Here's how the part is built. I have some questions about the finished solid (model axes, mm). Give positions to 0.01 mm unless a question says otherwise; leave off trailing zeros. Loops run counter-clockwise (first coordinate to the right, second up) from the corner with the lowest first, then second, coordinate; pieces in that order, holes last. Notation, with made-up numbers: (67.5, 26) - (119.5, 26) arc R21 cw to (119.5, 38) - close; hole circle Ø9 at (56, 71.5). An arc over 180 degrees is marked (long way). Return JSON: item names as keys, results as strings. Group by question number.
(1) If we section it at A-A (x = 149): Please give me the cut outline in (y, z) (1 decimal), then the cut area to 3 significant figures.
(2) I need wall thicknesses on probe 1 along X at (y, z) = (0.25, -214); probe 2 along Z at (x, y) = (221.5, -2). Which ranges of each line are inside material? Lowest first, please. Write a range as [from, to].
(3) If we section it at C-C (y = -0.5): State how many separate pieces and enclosed holes the cut face has, then the cut area to 3 significant figures.
(4) If we section it at B-B (z = -136): Please give me the cut outline in (x, y) (1 decimal), then the cut area to 3 significant figures.
```python
from build123d import *

# Parameters (mm, degrees)
SKETCH1_W                              = 382.775
SKETCH1_H                              = 356.150000032
BOSS_EXTRUDE1_DEPTH                    = 3.175
OUTER_SIDE_WALL_WELD_TAB_CUTOUTS_DEPTH = 6.35
CUT_EXTRUDE2_DEPTH                     = 6.35
CUT_EXTRUDE3_DEPTH                     = 6.35


with BuildPart() as part:
    # Sketch1 → Boss-Extrude1 (new body, symmetric)
    with BuildSketch(Plane(origin=(0, 0, 0), x_dir=(1, 0, 0), z_dir=(0, 1, 0))):
        with Locations((158.05, 144.737500016)):
            Rectangle(SKETCH1_W, SKETCH1_H)
    extrude(amount=BOSS_EXTRUDE1_DEPTH, both=True)

    # Sketch3 → Outer Side Wall Weld Tab Cutouts (cut)
    with BuildSketch(Plane(origin=(0, -3.175, 0), x_dir=(1, 0, 0), z_dir=(0, 1, 0))):
        with BuildLine():
            Line((314.5125, 53.318750008), (314.5125, 91.418750008))
            ThreePointArc((314.5125, 91.418750008), (316.1, 93.006250008), (317.6875, 91.418750008))
            Line((317.6875, 91.418750008), (317.6875, 53.318750008))
            ThreePointArc((317.6875, 53.318750008), (316.1, 51.731250008), (314.5125, 53.318750008))
        make_face()
        with BuildLine():
            Line((-1.5875, 53.318750008), (-1.5875, 91.418750008))
            ThreePointArc((-1.5875, 91.418750008), (0, 93.006250008), (1.5875, 91.418750008))
            Line((1.5875, 91.418750008), (1.5875, 53.318750008))
            ThreePointArc((1.5875, 53.318750008), (0, 51.731250008), (-1.5875, 53.318750008))
        make_face()
        with BuildLine():
            Line((314.5125, 125.687500016), (314.5125, 163.787500016))
            ThreePointArc((314.5125, 163.787500016), (316.1, 165.375000016), (317.6875, 163.787500016))
            Line((317.6875, 163.787500016), (317.6875, 125.687500016))
            ThreePointArc((317.6875, 125.687500016), (316.1, 124.100000016), (314.5125, 125.687500016))
        make_face()
        with BuildLine():
            Line((314.5125, 198.056250024), (314.5125, 236.156250024))
            ThreePointArc((314.5125, 236.156250024), (316.1, 237.743750024), (317.6875, 236.156250024))
            Line((317.6875, 236.156250024), (317.6875, 198.056250024))
            ThreePointArc((317.6875, 198.056250024), (316.1, 196.468750024), (314.5125, 198.056250024))
        make_face()
        with BuildLine():
            Line((-1.5875, 125.687500016), (-1.5875, 163.787500016))
            ThreePointArc((-1.5875, 163.787500016), (0, 165.375000016), (1.5875, 163.787500016))
            Line((1.5875, 163.787500016), (1.5875, 125.687500016))
            ThreePointArc((1.5875, 125.687500016), (0, 124.100000016), (-1.5875, 125.687500016))
        make_face()
        with BuildLine():
            Line((-1.5875, 198.056250024), (-1.5875, 236.156250024))
            ThreePointArc((-1.5875, 236.156250024), (0, 237.743750024), (1.5875, 236.156250024))
            Line((1.5875, 236.156250024), (1.5875, 198.056250024))
            ThreePointArc((1.5875, 198.056250024), (0, 196.468750024), (-1.5875, 198.056250024))
        make_face()
    extrude(amount=OUTER_SIDE_WALL_WELD_TAB_CUTOUTS_DEPTH, mode=Mode.SUBTRACT)

    # Sketch4 → Cut-Extrude2 (cut)
    with BuildSketch(Plane(origin=(0, -3.175, 0), x_dir=(1, 0, 0), z_dir=(0, 1, 0))):
        with BuildLine():
            Line((156.4625, 53.318750008), (156.4625, 91.418750008))
            ThreePointArc((156.4625, 91.418750008), (158.05, 93.006250008), (159.6375, 91.418750008))
            Line((159.6375, 91.418750008), (159.6375, 53.318750008))
            ThreePointArc((159.6375, 53.318750008), (158.05, 51.731250008), (156.4625, 53.318750008))
        make_face()
        with BuildLine():
            Line((77.4375, 53.318750008), (77.4375, 91.418750008))
            ThreePointArc((77.4375, 91.418750008), (79.025, 93.006250008), (80.6125, 91.418750008))
            Line((80.6125, 91.418750008), (80.6125, 53.318750008))
            ThreePointArc((80.6125, 53.318750008), (79.025, 51.731250008), (77.4375, 53.318750008))
        make_face()
        with BuildLine():
            Line((235.4875, 53.318750008), (235.4875, 91.418750008))
            ThreePointArc((235.4875, 91.418750008), (237.075, 93.006250008), (238.6625, 91.418750008))
            Line((238.6625, 91.418750008), (238.6625, 53.318750008))
            ThreePointArc((238.6625, 53.318750008), (237.075, 51.731250008), (235.4875, 53.318750008))
        make_face()
        with BuildLine():
            Line((156.4625, 125.687500016), (156.4625, 163.787500016))
            ThreePointArc((156.4625, 163.787500016), (158.05, 165.375000016), (159.6375, 163.787500016))
            Line((159.6375, 163.787500016), (159.6375, 125.687500016))
            ThreePointArc((159.6375, 125.687500016), (158.05, 124.100000016), (156.4625, 125.687500016))
        make_face()
        with BuildLine():
            Line((235.4875, 125.687500016), (235.4875, 163.787500016))
            ThreePointArc((235.4875, 163.787500016), (237.075, 165.375000016), (238.6625, 163.787500016))
            Line((238.6625, 163.787500016), (238.6625, 125.687500016))
            ThreePointArc((238.6625, 125.687500016), (237.075, 124.100000016), (235.4875, 125.687500016))
        make_face()
        with BuildLine():
            Line((156.4625, 198.056250024), (156.4625, 236.156250024))
            ThreePointArc((156.4625, 236.156250024), (158.05, 237.743750024), (159.6375, 236.156250024))
            Line((159.6375, 236.156250024), (159.6375, 198.056250024))
            ThreePointArc((159.6375, 198.056250024), (158.05, 196.468750024), (156.4625, 198.056250024))
        make_face()
        with BuildLine():
            Line((235.4875, 198.056250024), (235.4875, 236.156250024))
            ThreePointArc((235.4875, 236.156250024), (237.075, 237.743750024), (238.6625, 236.156250024))
            Line((238.6625, 236.156250024), (238.6625, 198.056250024))
            ThreePointArc((238.6625, 198.056250024), (237.075, 196.468750024), (235.4875, 198.056250024))
        make_face()
        with BuildLine():
            Line((77.4375, 125.687500016), (77.4375, 163.787500016))
            ThreePointArc((77.4375, 163.787500016), (79.025, 165.375000016), (80.6125, 163.787500016))
            Line((80.6125, 163.787500016), (80.6125, 125.687500016))
            ThreePointArc((80.6125, 125.687500016), (79.025, 124.100000016), (77.4375, 125.687500016))
        make_face()
        with BuildLine():
            Line((77.4375, 198.056250024), (77.4375, 236.156250024))
            ThreePointArc((77.4375, 236.156250024), (79.025, 237.743750024), (80.6125, 236.156250024))
            Line((80.6125, 236.156250024), (80.6125, 198.056250024))
            ThreePointArc((80.6125, 198.056250024), (79.025, 196.468750024), (77.4375, 198.056250024))
        make_face()
    extrude(amount=CUT_EXTRUDE2_DEPTH, mode=Mode.SUBTRACT)

    # Sketch5 → Cut-Extrude3 (cut)
    with BuildSketch(Plane(origin=(0, -3.175, 0), x_dir=(1, 0, 0), z_dir=(0, 1, 0))):
        with BuildLine():
            Line((139, 1.5875), (177.1, 1.5875))
            ThreePointArc((177.1, 1.5875), (178.6875, 0), (177.1, -1.5875))
            Line((177.1, -1.5875), (139, -1.5875))
            ThreePointArc((139, -1.5875), (137.4125, 0), (139, 1.5875))
        make_face()
        with BuildLine():
            Line((59.975, 1.5875), (98.075, 1.5875))
            ThreePointArc((98.075, 1.5875), (99.6625, 0), (98.075, -1.5875))
            Line((98.075, -1.5875), (59.975, -1.5875))
            ThreePointArc((59.975, -1.5875), (58.3875, 0), (59.975, 1.5875))
        make_face()
        with BuildLine():
            Line((218.025, 1.5875), (256.125, 1.5875))
            ThreePointArc((256.125, 1.5875), (257.7125, 0), (256.125, -1.5875))
            Line((256.125, -1.5875), (218.025, -1.5875))
            ThreePointArc((218.025, -1.5875), (216.4375, 0), (218.025, 1.5875))
        make_face()
        with BuildLine():
            Line((139, 291.062500032), (177.1, 291.062500032))
            ThreePointArc((177.1, 291.062500032), (178.6875, 289.475000032), (177.1, 287.887500032))
            Line((177.1, 287.887500032), (139, 287.887500032))
            ThreePointArc((139, 287.887500032), (137.4125, 289.475000032), (139, 291.062500032))
        make_face()
        with BuildLine():
            Line((218.025, 291.062500032), (256.125, 291.062500032))
            ThreePointArc((256.125, 291.062500032), (257.7125, 289.475000032), (256.125, 287.887500032))
            Line((256.125, 287.887500032), (218.025, 287.887500032))
            ThreePointArc((218.025, 287.887500032), (216.4375, 289.475000032), (218.025, 291.062500032))
        make_face()
        with BuildLine():
            Line((59.975, 291.062500032), (98.075, 291.062500032))
            ThreePointArc((98.075, 291.062500032), (99.6625, 289.475000032), (98.075, 287.887500032))
            Line((98.075, 287.887500032), (59.975, 287.887500032))
            ThreePointArc((59.975, 287.887500032), (58.3875, 289.475000032), (59.975, 291.062500032))
        make_face()
    extrude(amount=CUT_EXTRUDE3_DEPTH, mode=Mode.SUBTRACT)


solid = part.part
```
Values:
{
 "1": {"outline": "(-3.2, -322.8) - (3.2, -322.8) - (3.2, -291.1) - (-3.2, -291.1) - close; (-3.2, -287.9) - (3.2, -287.9) - (3.2, -1.6) - (-3.2, -1.6) - close; (-3.2, 1.6) - (3.2, 1.6) - (3.2, 33.3) - (-3.2, 33.3) - close", "area": "2,220 mm2"},
 "2": {"probe 1": "[-33.34, -1.59], [1.59, 77.44], [80.61, 156.46], [159.64, 235.49], [238.66, 314.51], [317.69, 349.44]", "probe 2": "[-322.81, -291.06], [-287.89, -1.59], [1.59, 33.34]"},
 "3": {"separate pieces": "1", "enclosed holes": "21", "area": "134,000 mm2"},
 "4": {"outline": "(-33.3, -3.2) - (-1.6, -3.2) - (-1.6, 3.2) - (-33.3, 3.2) - close; (1.6, -3.2) - (77.4, -3.2) - (77.4, 3.2) - (1.6, 3.2) - close; (80.6, -3.2) - (156.5, -3.2) - (156.5, 3.2) - (80.6, 3.2) - close; (159.6, -3.2) - (235.5, -3.2) - (235.5, 3.2) - (159.6, 3.2) - close; (238.7, -3.2) - (314.5, -3.2) - (314.5, 3.2) - (238.7, 3.2) - close; (317.7, -3.2) - (349.4, -3.2) - (349.4, 3.2) - (317.7, 3.2) - close", "area": "2,330 mm2"}
}
